from build123d import *

# Parameters (mm, degrees)
CROQUIS1_R              = 2.5
SALIENTE_EXTRUIR1_DEPTH = 10
CROQUIS2_W              = 83.7
CROQUIS2_H              = 12
SALIENTE_EXTRUIR2_DEPTH = 45
CROQUIS3_W              = 83.7
CROQUIS3_H              = 8
SALIENTE_EXTRUIR3_DEPTH = 10
CORTAR_EXTRUIR1_REACH   = 87.411
CROQUIS4_R              = 2.5


with BuildPart() as part:
    # Croquis1 → Saliente-Extruir1 (new body)
    with BuildSketch(Plane.XY):
        Polygon((-33.081084665, 4.522845957), (-33.081084665, -3.763368441), (50.618915335, -3.763368441), (50.618915335, 4.522845957), (50.618915335, 50.236631559), (-33.081084665, 50.236631559), (-33.081084665, 7.26530538), align=None)
        with Locations((-24.981084665, 14.486631559)):
            Circle(CROQUIS1_R, mode=Mode.SUBTRACT)
        with Locations(Location((-24.981084665, 31.986631559, 0), (0, 0, 180))):
            Circle(CROQUIS1_R, mode=Mode.SUBTRACT)
        with Locations((42.518915335, 31.986631559)):
            Circle(CROQUIS1_R, mode=Mode.SUBTRACT)
        with Locations(Location((42.518915335, 14.486631559, 0), (0, 0, 180))):
            Circle(CROQUIS1_R, mode=Mode.SUBTRACT)
        with BuildLine():
            Line((38.618915335, 38.236631559), (-21.081084665, 38.236631559))
            Line((-21.081084665, 38.236631559), (-21.081084665, 26.736631559))
            Line((-21.081084665, 26.736631559), (-24.681084665, 26.736631559))
            ThreePointArc((-24.681084665, 26.736631559), (-28.281084665, 23.236631559), (-24.681084665, 19.736631559))
            Line((-24.681084665, 19.736631559), (-21.081084665, 19.736631559))
            Line((-21.081084665, 19.736631559), (-21.081084665, 8.236631559))
            Line((-21.081084665, 8.236631559), (15.848469228, 8.236631559))
            Line((15.848469228, 8.236631559), (38.618915335, 8.236631559))
            Line((38.618915335, 8.236631559), (38.618915335, 38.236631559))
        make_face(mode=Mode.SUBTRACT)
    extrude(amount=SALIENTE_EXTRUIR1_DEPTH)

    # Croquis2 → Saliente-Extruir2 (add)
    with BuildSketch(Plane.XY.offset(10)):
        with Locations((8.768915335, 2.236631559)):
            Rectangle(CROQUIS2_W, CROQUIS2_H)
        with Locations((8.768915335, 44.236631559)):
            Rectangle(CROQUIS2_W, CROQUIS2_H)
    extrude(amount=SALIENTE_EXTRUIR2_DEPTH)

    # Croquis3 → Saliente-Extruir3 (add)
    with BuildSketch(Plane.XZ.offset(3.763368441)):
        with Locations((8.768915335, 51)):
            Rectangle(CROQUIS3_W, CROQUIS3_H)
    saliente_extruir3 = extrude(amount=SALIENTE_EXTRUIR3_DEPTH)

    # Croquis4 → Cortar-Extruir1 (cut, up to next)
    with BuildSketch(Plane(origin=(0, 0, 47), x_dir=(-1, 0, 0), z_dir=(0, 0, -1)), mode=Mode.PRIVATE) as cortar_extruir1_sk1:
        with Locations((-41.410138607, -8.763368441)):
            Circle(CROQUIS4_R)
    cortar_extruir1_tool1 = extrude(cortar_extruir1_sk1.sketch, amount=-CORTAR_EXTRUIR1_REACH, mode=Mode.PRIVATE) & part.part
    # Croquis4 → Cortar-Extruir1 (cut, up to next)
    with BuildSketch(Plane(origin=(0, 0, 47), x_dir=(-1, 0, 0), z_dir=(0, 0, -1)), mode=Mode.PRIVATE) as cortar_extruir1_sk2:
        with Locations(Location((23.872307937, -8.763368441, 0), (0, 0, 180))):
            Circle(CROQUIS4_R)
    cortar_extruir1_tool2 = extrude(cortar_extruir1_sk2.sketch, amount=-CORTAR_EXTRUIR1_REACH, mode=Mode.PRIVATE) & part.part
    cortar_extruir1_1 = cortar_extruir1_tool1.solids().sort_by_distance((41.410139, -8.763368, 47))[0]
    add(cortar_extruir1_1, mode=Mode.SUBTRACT)
    cortar_extruir1_2 = cortar_extruir1_tool2.solids().sort_by_distance((-23.872308, -8.763368, 47))[0]
    add(cortar_extruir1_2, mode=Mode.SUBTRACT)
    cortar_extruir1 = cortar_extruir1_1 + cortar_extruir1_2  # Cortar-Extruir1 as one shape, for the pattern or mirror that repeats it

    # Simetría1: Saliente-Extruir3, Cortar-Extruir1 across plane
    add(saliente_extruir3.mirror(Plane.ZX.offset(23.236631559)))
    add(cortar_extruir1.mirror(Plane.ZX.offset(23.236631559)), mode=Mode.SUBTRACT)


solid = part.part
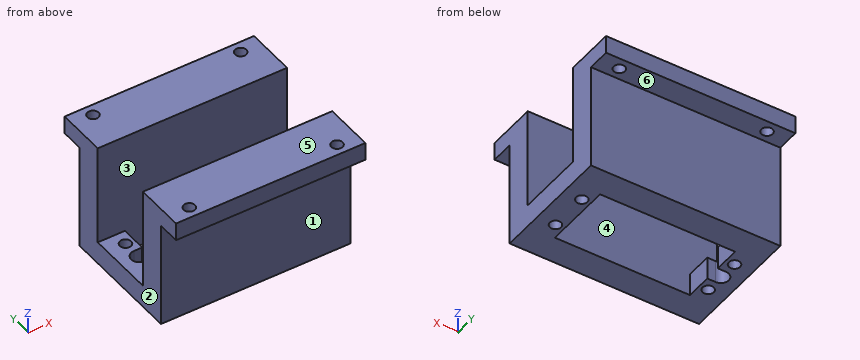
Source: CAD feature listing. Evaluate the final solid. Frame: model axes, mm. Face numbers are marked on the shaded views. A direction names the side the tool comes from. Give positions to 0.01 mm unless a question says otherwise; leave off trailing zeros. Loops run counter-clockwise (first coordinate to the right, second up) from the corner with the lowest first, then second, coordinate; pieces in that order, holes last. Notation, with made-up numbers: (52.25, 73.5) -> (100.25, 73.5) arc R25 ccw to (100.25, 90.5) -> close; hole circle Ø4 at (-31.75, -19.5). An arc over 180 degrees is marked (long way). Use a Markdown table: item, result. Add a question column.
1) Section query C-C, the plane y = 33. Return the cut outline in (x, z).
2) Section query D-D, the plane z = 6.5. Return the cut outline in (x, y).
3) Section query A-A, the plane x = 0. Return the cut outline in (y, z), then the cut area to 3 significant figures.
4) Reachability of the marked faces 4, 5 and 6 from +Z, -Z, +X, -X, +Y, -Y: full face, straight path, thin tool, end or side. Return the list, or none.
5) Pull-direction query (X, two-part tool) for the marked faces 1, 2 and 3; classes: +X half, -X half, draft (parallel to the pull), parting line (faces both ways), or undercut.
6) First-contact query: pin 1 (4 mm diameter, centred on x = -22, z = 6.5, fed in from +Y); pin 2 (14 mm diameter, centred on x = 9, z = 16.5, fed in from -Y); pin 3 (1 mm diameter, centred on x = 42, y = 34.5, fed in from +Z); pin 4 (3 mm diameter, centred on x = 42.52, y = 14.49, fed in from -Z). Flat tips, straight axial feed; report the tip coordinate or a pass-through.
7) Section query B-B, the plane z = 34.5. Return the cut outline in (x, y), then the cut area to 3 significant figures.
8) Line query: line 1 along Y through (x, z) = (-8.5, 42); line 2 along Y through (x, z) = (-19, 49); line 3 along Z through (x, y) = (-18, -4.5). Output: solid intervals per line, ascending. Write a range as [from, to].
Numbers:
| question | item | result |
|---|---|---|
| 1 | outline | (-33.08, 0) -> (-27.27, 0) -> (-27.27, 10) -> (-33.08, 10) -> close; (-22.7, 0) -> (-21.08, 0) -> (-21.08, 10) -> (-22.7, 10) -> close; (38.62, 0) -> (40.23, 0) -> (40.23, 10) -> (38.62, 10) -> close; (44.8, 0) -> (50.62, 0) -> (50.62, 10) -> (44.8, 10) -> close |
| 2 | outline | (-33.08, -3.76) -> (50.62, -3.76) -> (50.62, 50.24) -> (-33.08, 50.24) -> close; hole circle Ø5 at (-24.98, 14.49); hole circle Ø5 at (-24.98, 31.99); hole (-24.68, 19.74) -> (-21.08, 19.74) -> (-21.08, 8.24) -> (38.62, 8.24) -> (38.62, 38.24) -> (-21.08, 38.24) -> (-21.08, 26.74) -> (-24.68, 26.74) arc R3.5 ccw (long way) to start; hole circle Ø5 at (42.52, 14.49); hole circle Ø5 at (42.52, 31.99) |
| 3 | outline | (-13.76, 47) -> (-3.76, 47) -> (-3.76, 0) -> (8.24, 0) -> (8.24, 55) -> (-13.76, 55) -> close; (38.24, 0) -> (50.24, 0) -> (50.24, 47) -> (60.24, 47) -> (60.24, 55) -> (38.24, 55) -> close |
| 3 | area | 1,480 mm2 |
| 4 | face 4 | +Z |
| 4 | face 5 | +Z, +X, -X, +Y, -Y |
| 4 | face 6 | -Z, +X, -X, +Y |
| 5 | face 1 | draft |
| 5 | face 2 | -X half |
| 5 | face 3 | undercut |
| 6 | pin 1 | stops at y = 50.24 |
| 6 | pin 2 | stops at y = -3.76 |
| 6 | pin 3 | stops at z = 10 |
| 6 | pin 4 | passes through |
| 7 | outline | (-33.08, -3.76) -> (50.62, -3.76) -> (50.62, 8.24) -> (-33.08, 8.24) -> close; (-33.08, 38.24) -> (50.62, 38.24) -> (50.62, 50.24) -> (-33.08, 50.24) -> close |
| 7 | area | 2,010 mm2 |
| 8 | line 1 | y = [-3.76, 8.24], [38.24, 50.24] |
| 8 | line 2 | y = [-13.76, 8.24], [38.24, 60.24] |
| 8 | line 3 | z = [47, 55] |
